```python
from build123d import *

# Parameters (mm, degrees)
F1_DEPTH = 10
F3_DEPTH = 5
F5_DEPTH = 15
F8_DEPTH = 15
F9_DEPTH = 25


# Not quite as in the source:
# - a feature names something its author has since deleted; it is built from what else it names


with BuildPart() as f1:
    # F0 (on Front) → F1 (new body, symmetric)
    with BuildSketch(Plane.XZ):
        with BuildLine():
            Line((-62.5, -30), (-62.5, 0))
            Line((-62.5, 0), (-75, 0))
            ThreePointArc((-75, 0), (-73.4179734698, -15.3232232767), (-68.7386354243, -30))
            Line((-68.7386354243, -30), (-62.5, -30))
        make_face()
        with BuildLine():
            ThreePointArc((-68.7386354243, -30), (-73.4179734698, -15.3232232767), (-75, 0))
            Line((-75, 0), (-75, -30))
            Line((-75, -30), (-68.7386354243, -30))
        make_face()
        with BuildLine():
            Line((-75, 0), (-62.5, 0))
            ThreePointArc((-62.5, 0), (-44.1941738242, 44.1941738242), (0, 62.5))
            Line((0, 62.5), (0, 75))
            ThreePointArc((0, 75), (-53.033008589, 53.033008589), (-75, 0))
        make_face()
        with BuildLine():
            ThreePointArc((0, 62.5), (23.9177145228, 57.742470782), (44.1941738242, 44.1941738242))
            Line((44.1941738242, 44.1941738242), (44.1941738242, 56.6941738242))
            Line((44.1941738242, 56.6941738242), (49.0995993303, 56.6941738242))
            ThreePointArc((49.0995993303, 56.6941738242), (26.2005435362, 70.274686185), (0, 75))
            Line((0, 75), (0, 62.5))
        make_face()
        with BuildLine():
            Line((44.1941738242, 56.6941738242), (44.1941738242, 44.1941738242))
            Line((44.1941738242, 44.1941738242), (53.033008589, 53.033008589))
            ThreePointArc((53.033008589, 53.033008589), (51.0991040315, 54.8988302897), (49.0995993303, 56.6941738242))
            Line((49.0995993303, 56.6941738242), (44.1941738242, 56.6941738242))
        make_face()
        with BuildLine():
            ThreePointArc((49.0995993303, 56.6941738242), (51.0991040315, 54.8988302897), (53.033008589, 53.033008589))
            ThreePointArc((53.033008589, 53.033008589), (56.9861303035, 48.7604445533), (60.5959982177, 44.1941738242))
            Line((60.5959982177, 44.1941738242), (79.1941738242, 44.1941738242))
            Line((79.1941738242, 44.1941738242), (79.1941738242, 56.6941738242))
            Line((79.1941738242, 56.6941738242), (49.0995993303, 56.6941738242))
        make_face()
        with BuildLine():
            Line((53.033008589, 53.033008589), (44.1941738242, 44.1941738242))
            Line((44.1941738242, 44.1941738242), (60.5959982177, 44.1941738242))
            ThreePointArc((60.5959982177, 44.1941738242), (56.9861303035, 48.7604445533), (53.033008589, 53.033008589))
        make_face()
    extrude(amount=F1_DEPTH, both=True)

    # F2 (on Front) → F3 (cut, symmetric)
    with BuildSketch(Plane.XZ):
        with BuildLine():
            Line((45.9241320293, 52.8296706156), (49.2044271743, 56.6032185167))
            ThreePointArc((49.2044271743, 56.6032185167), (-31.1019931992, 68.2470953157), (-75, 0))
            Line((-75, 0), (-70, 0))
            ThreePointArc((-70, 0), (-29.0285269859, 63.6972889614), (45.9241320293, 52.8296706156))
        make_face()
    extrude(amount=F3_DEPTH, both=True, mode=Mode.SUBTRACT)


with BuildPart() as f5:
    # F4 (on Front) → F5 (new body)
    with BuildSketch(Plane.XZ):
        with BuildLine():
            ThreePointArc((-56.6264457982, 9.9847702158), (-36.960287557, 44.0475554793), (0, 57.5))
            Line((0, 57.5), (0, 80))
            ThreePointArc((0, 80), (-51.4230087749, 61.2835554495), (-78.784620241, 13.8918542134))
            Line((-78.784620241, 13.8918542134), (-56.6264457982, 9.9847702158))
        make_face()
    extrude(amount=F5_DEPTH)

    # F6: cut F1
    add(f1.part, mode=Mode.SUBTRACT)

    # F7 (on face) → F8 (join, through all)
    with BuildSketch(Plane.XZ.offset(15)):
        with BuildLine():
            ThreePointArc((-47.389204942, 32.5655224887), (-48.6302678935, 30.6813794443), (-49.7964607176, 28.75))
            Line((-49.7964607176, 28.75), (-45.4663336987, 26.25))
            ThreePointArc((-45.4663336987, 26.25), (-44.4015489462, 28.0134334057), (-43.2684045123, 29.7337379245))
            Line((-43.2684045123, 29.7337379245), (-47.389204942, 32.5655224887))
        make_face()
        with BuildLine():
            Line((-14.4709611804, 50.4662390368), (-15.8491479595, 55.2725475165))
            ThreePointArc((-15.8491479595, 55.2725475165), (-17.7684771766, 54.685749687), (-19.6661582412, 54.0323256952))
            Line((-19.6661582412, 54.0323256952), (-17.9560575246, 49.3338625913))
            ThreePointArc((-17.9560575246, 49.3338625913), (-16.2233922047, 49.9304671055), (-14.4709611804, 50.4662390368))
        make_face()
    extrude(amount=-F8_DEPTH)

    # F7 (on face) → F9 (cut)
    with BuildSketch(Plane.XZ.offset(15)):
        with BuildLine():
            Line((-48.9153382675, 38.9042373293), (-45.0021112061, 35.7918983429))
            ThreePointArc((-45.0021112061, 35.7918983429), (-43.7255778977, 37.3406459172), (-42.395771708, 38.8438996663))
            Line((-42.395771708, 38.8438996663), (-46.0823605522, 42.221630072))
            ThreePointArc((-46.0823605522, 42.221630072), (-47.5278020627, 40.5876586056), (-48.9153382675, 38.9042373293))
        make_face()
        with BuildLine():
            ThreePointArc((-11.3558821654, 56.3674901006), (-9.3817674339, 56.7294671209), (-7.396222464, 57.0223280239))
            Line((-7.396222464, 57.0223280239), (-8.0393722435, 61.9807913303))
            ThreePointArc((-8.0393722435, 61.9807913303), (-10.1975732978, 61.6624642618), (-12.3433501798, 61.269010979))
            Line((-12.3433501798, 61.269010979), (-11.3558821654, 56.3674901006))
        make_face()
    extrude(amount=-F9_DEPTH, mode=Mode.SUBTRACT)


solid = f5.part
```
Work out the finished part from the listing and answer in its coordinate system (mm). A direction names the side the tool comes from. Give positions to 0.01 mm unless a question says otherwise; leave off trailing zeros. Loops run counter-clockwise (first coordinate to the right, second up) from the corner with the lowest first, then second, coordinate; pieces in that order, holes last. Notation, with made-up numbers: (-24.5, 64.5) -> (10.5, 64.5) arc R26 ccw to (10.5, 101.5) -> close; hole circle Ø8 at (38, 49). An arc over 180 degrees is marked (long way). One line per question, with ' | ' between items. Start each with the question number.
1) Determine the mould class of faces 1 (the face through (-67.861, -10.728, 11.966)), 2 (the face through (-45.3, -7.6, 31.13)), 3 (the face through (-7.713, -7.605, 59.467)) for opening direction X: +X half, -X half, draft (parallel to the pull), parting line (faces both ways), or undercut.
2) Straight lines are drawn through the part: L1, parallel to X at y = -6.5, z = 28.5; L2, parallel to X at y = -5.25, z = 33.5; L3, parallel to Z at x = -48, y = -9.5. For each, find the intervals that lie inside material, in ascending order.
3) Each of these flat-tipped pins is pushed along its axis until it touches: pin 1 (3 mm diameter, centred on y = -2, z = 26.5, fed in from -X); pin 2 (2 mm diameter, centred on y = -5.5, z = 47, fed in from -X); pin 3 (3 mm diameter, centred on y = -11, z = 30.5, fed in from +X); pin 4 (8 mm diameter, centred on x = -45.5, z = 29.5, fed in from +Y). Where does it stop, or does it pass through?
4) Section B-B, the plane z = 52 is taken. Determine the outline of the cut face in (x, y), then the cut area to 3 significant figures.
5) Section A-A, the plane y = -1 is taken. Determine the outline of the cut face in (x, z).
6) Section D-D, the plane x = -37 is taken. Determine the outline of the cut face in (y, z), then the cut area to 3 significant figures.
7) For faces 4 (the face through (-4.084, -5.07, 62.366)), 5 (the face through (-45, -5, 55)), 6 (the face through (-46.24, -7.4, 34.18)), determine the directions among +Z, -Z, +X, -X, +Y, -Y from which every point of the face is accessible in a straight line to the end or side of a thin tool.
8) Section C-C, the plane y = -12 is taken. Determine the outline of the cut face in (x, z), then the cut area to 3 significant figures.
Resolved:
1) face 1: -X half | face 2: +X half | face 3: undercut
2) L1: -74.75 to -69.37, -55.62 to -49.94, -49.36 to -44.09 | L2: -72.65 to -67.1, -52.76 to -46.73 | L3: 27.71 to 38.18, 57.63 to 64
3) pin 1: x = -75.99 | pin 2: x = -65.45 | pin 3: x = -43.27 | pin 4: y = 0
4) outline: (-60.79, -15) -> (-24.54, -15) -> (-24.54, 0) -> (-34.67, 0) -> (-34.67, -10) -> (-54.05, -10) -> (-54.05, -5) -> (-46.86, -5) -> (-46.86, 0) -> (-60.79, 0) -> close; (-18.93, -15) -> (-14.91, -15) -> (-14.91, 0) -> (-18.93, 0) -> close | area: 446 mm2
5) outline: (-78.78, 13.89) -> (-68.94, 12.16) arc R70 cw to (0, 70) -> (0, 80) arc R80 ccw to start; (-61.55, 10.85) -> (-56.63, 9.98) arc R57.5 cw to (-49.8, 28.75) -> (-45.47, 26.25) arc R52.5 cw to (-43.27, 29.73) -> (-47.39, 32.57) arc R57.5 cw to (-45, 35.79) -> (-48.92, 38.9) arc R62.5 ccw to start; (-46.08, 42.22) -> (-42.4, 38.84) arc R57.5 cw to (-19.67, 54.03) -> (-17.96, 49.33) arc R52.5 cw to (-14.47, 50.47) -> (-15.85, 55.27) arc R57.5 cw to (-11.36, 56.37) -> (-12.34, 61.27) arc R62.5 ccw to start; (-8.04, 61.98) -> (-7.4, 57.02) arc R57.5 cw to (0, 57.5) -> (0, 62.5) arc R62.5 ccw to start
6) outline: (-15, 44.01) -> (0, 44.01) -> (0, 50.37) -> (-10, 50.37) -> (-10, 65.24) -> (-5, 65.24) -> (-5, 59.42) -> (0, 59.42) -> (0, 70.93) -> (-15, 70.93) -> close | area: 284 mm2
7) face 4: +Y | face 5: none | face 6: +X, +Y, -Y
8) outline: (-78.78, 13.89) -> (-56.63, 9.98) arc R57.5 cw to (-49.8, 28.75) -> (-45.47, 26.25) arc R52.5 cw to (-43.27, 29.73) -> (-47.39, 32.57) arc R57.5 cw to (-45, 35.79) -> (-48.92, 38.9) arc R62.5 cw to (-46.08, 42.22) -> (-42.4, 38.84) arc R57.5 cw to (-19.67, 54.03) -> (-17.96, 49.33) arc R52.5 cw to (-14.47, 50.47) -> (-15.85, 55.27) arc R57.5 cw to (-11.36, 56.37) -> (-12.34, 61.27) arc R62.5 cw to (-8.04, 61.98) -> (-7.4, 57.02) arc R57.5 cw to (0, 57.5) -> (0, 80) arc R80 ccw to start | area: 2,160 mm2
